Check sheet for the modelled part. Datum: model origin and axes. Units: mm. A direction names the side the tool comes from. Give positions to 0.01 mm unless a question says otherwise; leave off trailing zeros. Order: outer loops, then holes, each group sorted by start corner. A loop starts at its lowest first (then second) coordinate and runs counter-clockwise, first axis right, second up. Notation, with made-up numbers: M -40,62.25 L 18,62.25 A15 cw 18,78.25 Z; hole C 70,78 d10. An arc over 180 degrees is marked long. Return JSON: item names as keys, results as strings. Group by question number.
from build123d import *

# Parameters (mm, degrees)
F0_W     = 50.8
F0_H     = 15.24
F1_DEPTH = 9.525
F2_R     = 2.159
F3_DEPTH = 11.1125
F4_R     = 2.032
F5_R     = 5.08


with BuildPart() as f1:
    # F0 (on Top) → F1 (new body)
    with BuildSketch(Plane.XY):
        Rectangle(F0_W, F0_H)
    extrude(amount=F1_DEPTH)

    # F2 (on face) → F3 (join)
    with BuildSketch(Plane.XY.offset(9.525)):
        with Locations((-19.05, 0)):
            Circle(F2_R)
        with Locations((19.05, 0)):
            Circle(F2_R)
    extrude(amount=F3_DEPTH)

    # F4
    f4_edges = [f1.edges().sort_by_distance(p)[0] for p in [
        (-21.209, 0, 20.6375),
        (16.891, 0, 20.6375),
    ]]
    fillet(f4_edges, radius=F4_R)

    # F5
    f5_edges = [f1.edges().sort_by_distance(p)[0] for p in [
        (-25.4, -7.62, 4.7625),
        (25.4, -7.62, 4.7625),
        (25.4, 7.62, 4.7625),
        (-25.4, 7.62, 4.7625),
    ]]
    fillet(f5_edges, radius=F5_R)


solid = f1.part
1) Material ranges on line 1 along Z through (x, y) = (-15, -4) (3 decimals); line 2 along X through (y, z) = (-6.25, 6.5); line 3 along X through (y, z) = (4.75, 3), recorded low to high.
2) Release check for a two-part mould opening along X. For faces 1 (the face through (0, 0, 9.525)), 2 (the face through (0, 7.62, 5)), 3 (the face through (-23.951, -6.092, 4.829)) record: released by +X, released by -X, zero draft, split by the parting line, or undercut.
3) Sectioned sample at D-D on y = 5.75. Record the boundary of the cut face in (x, z) (3 decimals), then the cut area to 3 significant figures.
4) Sectioned sample at C-C on x = 22.5. Record the boundary of the cut face in (y, z) (3 decimals).
5) Tool access check on faces 4 (the face through (17.337, -1.314, 14.002)), 5 (the face through (23.872, -6.171, 4.829)). Record the directions out of +Z, -Z, +X, -X, +Y, -Y that give a thin tool (end or side, any length) a straight path to the whole face; none if there is none.
6) Sectioned sample at B-B on z = 1.5. Record the boundary of the cut face in (x, y), then the cut area to 3 significant figures.
7) Sectioned sample at A-A on z = 14. Record the boundary of the cut face in (x, y), then the cut area to 3 significant figures.
8) Depth check by flat-ended pin: P1, Ø1.5, axis at y = -4, z = 16.5, coming from the +X side; P2, Ø4.5, axis at x = 10, y = -2.5, coming from the +Z side (3 decimals); P3, Ø6, axis at y = -0.5, z = 13, coming from the +X side; P4, Ø3, axis at y = 3, z = 16.5, coming from the -X side. Enter the tip coordinate at first touch or a pass-through.
Reply:
{
 "1": {"line 1": "0 to 9.525", "line 2": "-23.79 to 23.79", "line 3": "-24.89 to 24.89"},
 "2": {"face 1": "undercut", "face 2": "zero draft", "face 3": "released by -X"},
 "3": {"outline": "M -24.257,0 L 24.257,0 L 24.257,9.525 L -24.257,9.525 Z", "area": "462 mm^2"},
 "4": {"outline": "M -7.128,0 L 7.128,0 L 7.128,9.525 L -7.128,9.525 Z"},
 "5": {"face 4": "+Z", "face 5": "+Z, -Z, +X, -Y"},
 "6": {"outline": "M -25.4,-2.54 A5.08 ccw -20.32,-7.62 L 20.32,-7.62 A5.08 ccw 25.4,-2.54 L 25.4,2.54 A5.08 ccw 20.32,7.62 L -20.32,7.62 A5.08 ccw -25.4,2.54 Z", "area": "752 mm^2"},
 "7": {"outline": "C -19.05,0 d4.32; C 19.05,0 d4.32", "area": "29.3 mm^2"},
 "8": {"P1": "through", "P2": "z = 9.525", "P3": "x = 21.21", "P4": "x = -20.6"}
}
